```python
from build123d import *

# Parameters (mm, degrees)
SKETCH_1_R               = 11
EXTRUDE_1_DEPTH          = 8
FILLET_1_R               = 100
EXTRUDE_2_DEPTH          = 10
FILLET_2_R               = 10
CHAMFER_1_SIZE           = 5
SKETCH_4_R               = 13
CUT_EXTRUDE_1_DEPTH      = 0.7
SKETCH_5_R               = 2.5
CUT_EXTRUDE_2_DEPTH      = 434.184093957
SKETCH_6_R               = 6
CUT_EXTRUDE_3_DEPTH      = 4
CUT_EXTRUDE_4_DEPTH      = 434.442567426
CUT_EXTRUDE_4_DEPTH_BACK = 434.442567426
SKETCH_7_R               = 4.3


with BuildPart() as part:
    # Sketch 1 → Extrude 1 (new body)
    with BuildSketch(Plane.XY):
        Polygon((0, 0), (0, 280), (861.751390409, 0), align=None)
        with Locations((200, 100)):
            Circle(SKETCH_1_R, mode=Mode.SUBTRACT)
    extrude(amount=EXTRUDE_1_DEPTH)

    # Fillet 1
    fillet_1_edges = [part.edges().sort_by_distance(p)[0] for p in [
        (861.751390409, 0, 4),
    ]]
    fillet(fillet_1_edges, radius=FILLET_1_R)

    # Sketch 2 → Extrude 2 (add)
    with BuildSketch(Plane.XY):
        with BuildLine():
            Line((0, 0), (230.376238942, 0))
            ThreePointArc((230.376238942, 0), (329.145073001, 84.356553496), (261.277938379, 195.10565163))
            Line((261.277938379, 195.10565163), (0, 280))
            Line((0, 280), (0, 0))
        make_face()
        Polygon((10, 266.236180795), (10, 35.358983849), (122.241374643, 229.766747442), align=None, mode=Mode.SUBTRACT)
        with BuildLine():
            Line((30, 10), (230.376238942, 10))
            ThreePointArc((230.376238942, 10), (319.268189595, 85.920898146), (258.187768435, 185.595086467))
            Line((258.187768435, 185.595086467), (151.410485182, 220.289128906))
            Line((151.410485182, 220.289128906), (30, 10))
        make_face(mode=Mode.SUBTRACT)
    extrude(amount=-EXTRUDE_2_DEPTH)

    # Fillet 2
    fillet_2_edges = [part.edges().sort_by_distance(p)[0] for p in [
        (30, 10, -5),
        (10, 266.236180795, -5),
        (10, 35.358983849, -5),
        (122.241374643, 229.766747442, -5),
        (151.410485182, 220.289128906, -5),
    ]]
    fillet(fillet_2_edges, radius=FILLET_2_R)

    # Chamfer 1
    chamfer_1_edges = [part.edges().sort_by_distance(p)[0] for p in [
        (130.63896919, 237.552825815, 8),
        (329.145073001, 84.356553496, 8),
        (130.63896919, 237.552825815, -10),
        (329.145073001, 84.356553496, -10),
        (115.188119471, 0, -10),
        (115.188119471, 0, 8),
    ]]
    chamfer(chamfer_1_edges, length=CHAMFER_1_SIZE)

    # Sketch 4 → Cut-Extrude 1 (cut)
    with BuildSketch(Plane(origin=(0, 0, 0), x_dir=(-1, 0, 0), z_dir=(0, 0, -1))):
        with Locations((-200, 100)):
            Circle(SKETCH_4_R)
    extrude(amount=-CUT_EXTRUDE_1_DEPTH, mode=Mode.SUBTRACT)

    # Sketch 5 → Cut-Extrude 2 (cut, through all)
    with BuildSketch(Plane(origin=(0, 0, 0), x_dir=(-1, 0, 0), z_dir=(0, 0, -1))):
        with Locations((-200, 130)):
            Circle(SKETCH_5_R)
        with Locations((-200, 70)):
            Circle(SKETCH_5_R)
    extrude(amount=-CUT_EXTRUDE_2_DEPTH, mode=Mode.SUBTRACT)

    # Sketch 6 → Cut-Extrude 3 (cut)
    with BuildSketch(Plane.XY.offset(8)):
        with Locations((200, 130)):
            Circle(SKETCH_6_R)
        with Locations((200, 70)):
            Circle(SKETCH_6_R)
    extrude(amount=-CUT_EXTRUDE_3_DEPTH, mode=Mode.SUBTRACT)

    # Sketch 7 → Cut-Extrude 4 (cut, two sides: drawn at the far end of the back side and taken through both)
    with BuildSketch(Plane.XY.offset(8).offset(-CUT_EXTRUDE_4_DEPTH_BACK)):
        with Locations((64, 217)):
            Circle(SKETCH_7_R)
        with Locations((24, 217)):
            Circle(SKETCH_7_R)
        with Locations((64, 177)):
            Circle(SKETCH_7_R)
        with Locations((24, 177)):
            Circle(SKETCH_7_R)
        with Locations((64, 89)):
            Circle(SKETCH_7_R)
        with Locations((24, 89)):
            Circle(SKETCH_7_R)
        with Locations((64, 49)):
            Circle(SKETCH_7_R)
        with Locations((24, 49)):
            Circle(SKETCH_7_R)
    extrude(amount=CUT_EXTRUDE_4_DEPTH + CUT_EXTRUDE_4_DEPTH_BACK, mode=Mode.SUBTRACT)


solid = part.part
```
Verification items for the finished model (mm, model axes). A direction names the side the tool comes from. Give positions to 0.01 mm unless a question says otherwise; leave off trailing zeros. Order: outer loops, then holes, each group sorted by start corner. A loop starts at its lowest first (then second) coordinate and runs counter-clockwise, first axis right, second up. Notation, with made-up numbers: M 30,24.5 L 61,24.5 A8 cw 61,36.5 Z; hole C 54.25,69 d9. An arc over 180 degrees is marked long. Return JSON: item names as keys, results as strings. Group by question number.
1) Section check A-A on y = 100. Record the cut outline in (x, z).
2) Go/stop test with flat-tipped pins: pin 1 Ø4 at (x, z) = (225, -8) entering from -Y; pin 2 Ø10 at (x, y) = (24, 89) entering from -Z; pin 3 Ø9.5 at (x, y) = (199.5, 67.5) entering from +Z; pin 4 Ø15.5 at (x, y) = (200, 100) entering from -Z. Record where each tip stops, or that it passes through.
3) Section check C-C on y = 204. Record the cut outline in (x, z), and give its area (3 significant figures).
4) Access from +Z, -Z, +X, -X, +Y, -Y to the whole of each face (thin tool, end or side, straight path). Record for faces 1 (the face through (189, 100, 4)), 2 (the face through (194, 70, 6)), 3 (the face through (318.97, 84.16, -4.93)).
5) Mould release check, pull along Y, two halves, no side actions. Record for faces 4 (the face through (324.79, 86.96, 7.69)), 5 (the face through (0, 142, -1)), 6 (the face through (66.312, 92.626, -1.126)): pulls with the +Y half, pulls with the -Y half, needs draft (parallel to the pull), parting line crosses it, or undercut.
6) Section check D-D on y = 49. Give the number of separate pieces and of enclosed holes in the cut face, and give its area (3 significant figures).
7) Section check B-B on x = 134. Record the cut outline in (y, z), and give its area (3 significant figures).
8) Scan lines: line 1 (Y direction, x = 21.5, z = -5.5); line 2 (X direction, y = 118.5, z = -3); line 3 (Y direction, x = 64, z = -4). Record each from-to range of solid material in increasing order.
Answer block:
{
 "1": {"outline": "M 0,-10 L 10,-10 L 10,0 L 47.32,0 L 47.32,-10 L 81.96,-10 L 81.96,0 L 187,0 L 187,0.7 L 189,0.7 L 189,8 L 0,8 Z; M 211,0.7 L 213,0.7 L 213,0 L 320.38,0 L 320.38,-10 L 325.38,-10 L 330.38,-5 L 330.38,3 L 325.38,8 L 211,8 Z"},
 "2": {"pin 1": "stops at y = 1", "pin 2": "stops at z = 0", "pin 3": "stops at z = 8", "pin 4": "passes through"},
 "3": {"outline": "M 0,-10 L 10,-10 L 10,0 L 107.36,0 L 107.36,-10 L 142.01,-10 L 142.01,0 L 201.54,0 L 201.54,-10 L 217.72,-10 L 233.9,-5 L 233.9,3 L 217.72,8 L 0,8 Z", "area": "2,560 mm^2"},
 "4": {"face 1": "+Z, -Z", "face 2": "+Z", "face 3": "-Z"},
 "5": {"face 4": "parting line crosses it", "face 5": "needs draft", "face 6": "undercut"},
 "6": {"separate pieces": "3", "enclosed holes": "0", "area": "2,920 mm^2"},
 "7": {"outline": "M 0,-5 L 5,-10 L 10,-10 L 10,0 L 190.13,0 L 190.13,-10 L 231.2,-10 L 236.46,-5 L 236.46,3 L 231.2,8 L 5,8 L 0,3 Z", "area": "2,400 mm^2"},
 "8": {"line 1": "y = 0.5 to 45.5, 52.5 to 62.79, 262.36 to 272.49", "line 2": "x = 0 to 10, 58 to 92.64, 318.45 to 328.65", "line 3": "y = 0 to 10, 68.89 to 84.7, 93.3 to 128.89, 248.69 to 259.21"}
}
